from build123d import *

# Parameters (mm, degrees)
SKETCH_1_W          = 330
SKETCH_1_H          = 225
EXTRUDE_1_DEPTH     = 5
SKETCH_2_R          = 2
CUT_EXTRUDE_1_DEPTH = 395.101001153
SKETCH_3_R          = 2
CUT_EXTRUDE_2_DEPTH = 395.101001153
CUT_EXTRUDE_4_DEPTH = 395.101001153
SKETCH_6_R          = 2
CUT_EXTRUDE_5_DEPTH = 395.101001153


with BuildPart() as part:
    # 草图1 → 凸台-拉伸1 (new body)
    with BuildSketch(Plane(origin=(0, 0, 0), x_dir=(1, 0, 0), z_dir=(0, 1, 0))):
        with Locations((149.701456311, 124.678398058)):
            Rectangle(SKETCH_1_W, SKETCH_1_H)
    extrude(amount=EXTRUDE_1_DEPTH)

    # 草图2 → 切除-拉伸1 (cut, through all)
    with BuildSketch(Plane(origin=(0, 5, 0), x_dir=(1, 0, 0), z_dir=(0, 1, 0))):
        with Locations(Location((137.701456311, 230.178398058, 0), (0, 0, 270))):
            Circle(SKETCH_2_R)
        with Locations(Location((161.701456311, 230.178398058, 0), (0, 0, 90))):
            Circle(SKETCH_2_R)
        with Locations(Location((137.701456311, 212.178398058, 0), (0, 0, 270))):
            Circle(SKETCH_2_R)
        with Locations(Location((161.701456311, 212.178398058, 0), (0, 0, 90))):
            Circle(SKETCH_2_R)
        with BuildLine():
            Line((34.701456311, 225.715369926), (84.701456311, 225.715369926))
            ThreePointArc((84.701456311, 225.715369926), (89.238428179, 221.178398058), (84.701456311, 216.64142619))
            Line((84.701456311, 216.64142619), (34.701456311, 216.64142619))
            ThreePointArc((34.701456311, 216.64142619), (30.164484443, 221.178398058), (34.701456311, 225.715369926))
        make_face()
        with BuildLine():
            Line((264.701456311, 225.715369926), (214.701456311, 225.715369926))
            ThreePointArc((214.701456311, 225.715369926), (210.164484443, 221.178398058), (214.701456311, 216.64142619))
            Line((214.701456311, 216.64142619), (264.701456311, 216.64142619))
            ThreePointArc((264.701456311, 216.64142619), (269.238428179, 221.178398058), (264.701456311, 225.715369926))
        make_face()
    extrude(amount=-CUT_EXTRUDE_1_DEPTH, mode=Mode.SUBTRACT)

    # 草图3 → 切除-拉伸2 (cut, through all)
    with BuildSketch(Plane(origin=(0, 5, 0), x_dir=(1, 0, 0), z_dir=(0, 1, 0))):
        with Locations(Location((-0.298543689, 32.178398058, 0), (0, 0, 270))):
            Circle(SKETCH_3_R)
        with Locations(Location((-0.298543689, 72.178398058, 0), (0, 0, 90))):
            Circle(SKETCH_3_R)
        with Locations(Location((41.701456311, 32.178398058, 0), (0, 0, 270))):
            Circle(SKETCH_3_R)
        with Locations(Location((41.701456311, 72.178398058, 0), (0, 0, 90))):
            Circle(SKETCH_3_R)
        with Locations(Location((257.701456311, 72.178398058, 0), (0, 0, 270))):
            Circle(SKETCH_3_R)
        with Locations(Location((257.701456311, 32.178398058, 0), (0, 0, 90))):
            Circle(SKETCH_3_R)
        with Locations(Location((299.701456311, 72.178398058, 0), (0, 0, 270))):
            Circle(SKETCH_3_R)
        with Locations(Location((299.701456311, 32.178398058, 0), (0, 0, 90))):
            Circle(SKETCH_3_R)
    extrude(amount=-CUT_EXTRUDE_2_DEPTH, mode=Mode.SUBTRACT)

    # 草图5 → 切除-拉伸4 (cut, through all)
    with BuildSketch(Plane(origin=(0, 5, 0), x_dir=(1, 0, 0), z_dir=(0, 1, 0))):
        with BuildLine():
            Line((155.701456311, 161.411602286), (155.701456311, 61.411602286))
            ThreePointArc((155.701456311, 61.411602286), (149.701456311, 55.411602286), (143.701456311, 61.411602286))
            Line((143.701456311, 61.411602286), (143.701456311, 161.411602286))
            ThreePointArc((143.701456311, 161.411602286), (149.701456311, 167.411602286), (155.701456311, 161.411602286))
        make_face()
        with BuildLine():
            Line((239.701456311, 161.411602286), (239.701456311, 61.411602286))
            ThreePointArc((239.701456311, 61.411602286), (233.701456311, 55.411602286), (227.701456311, 61.411602286))
            Line((227.701456311, 61.411602286), (227.701456311, 161.411602286))
            ThreePointArc((227.701456311, 161.411602286), (233.701456311, 167.411602286), (239.701456311, 161.411602286))
        make_face()
        with BuildLine():
            Line((59.701456311, 161.411602286), (59.701456311, 61.411602286))
            ThreePointArc((59.701456311, 61.411602286), (65.701456311, 55.411602286), (71.701456311, 61.411602286))
            Line((71.701456311, 61.411602286), (71.701456311, 161.411602286))
            ThreePointArc((71.701456311, 161.411602286), (65.701456311, 167.411602286), (59.701456311, 161.411602286))
        make_face()
    extrude(amount=-CUT_EXTRUDE_4_DEPTH, mode=Mode.SUBTRACT)

    # 草图6 → 切除-拉伸5 (cut, through all)
    with BuildSketch(Plane(origin=(0, 5, 0), x_dir=(1, 0, 0), z_dir=(0, 1, 0))):
        with Locations(Location((1.226003167, 225.911661565, 0), (0, 0, 270))):
            Circle(SKETCH_6_R)
        with Locations(Location((298.176909455, 225.911661565, 0), (0, 0, 90))):
            Circle(SKETCH_6_R)
        with Locations(Location((69.701456311, 22.178398058, 0), (0, 0, 270))):
            Circle(SKETCH_6_R)
        with Locations(Location((229.701456311, 22.178398058, 0), (0, 0, 90))):
            Circle(SKETCH_6_R)
    extrude(amount=-CUT_EXTRUDE_5_DEPTH, mode=Mode.SUBTRACT)


solid = part.part
Verification items for the finished model (mm, model axes). A direction names the side the tool comes from. Coordinates: 2 decimals unless noted, no trailing zeros. Order: outer loops, then holes, each group sorted by start corner. A loop starts at its lowest first (then second) coordinate and runs counter-clockwise, first axis right, second up. Notation, with made-up numbers: M 61,38 L 76,38 A9 ccw 76,51 Z; hole C 0,7 d3. An arc over 180 degrees is marked long. Write each question's results on one line, items separated by ' | '.
1) Gauge pin test, flat end, axial feed: pin 1 Ø3 at (x, z) = (229.7, -22.18) entering from +Y. Record the tip position at first contact, or that the pin passes through.
Solved:
pin 1: passes through
2) Section check B-B on y = 1.3. Give the number of separate pieces and of enclosed holes in the cut face, plus the area to 3 significant figures.
Solved:
separate pieces: 1 | enclosed holes: 21 | area: 69,100 mm²
3) Access from +Z, -Z, +X, -X, +Y, -Y to the whole of each face (thin tool, end or side, straight path). Record for faces 1 (the face through (184, 0, -126)), 2 (the face through (65.83, 2.54, -167.41)).
Solved:
face 1: +Z, -Z, +X, -X, -Y | face 2: +Y, -Y
4) Scan lines: line 1 along X through (y, z) = (3.45, -117); line 2 along X through (y, z) = (0.65, -212.5); line 3 along Z through (x, y) = (237, 0.85). Record each from-to range of solid material in increasing order. Write a range as [from, to].
Solved:
line 1: x = [-15.3, 59.7], [71.7, 143.7], [155.7, 227.7], [239.7, 314.7] | line 2: x = [-15.3, 135.73], [139.68, 159.73], [163.68, 314.7] | line 3: z = [-237.18, -225.72], [-216.64, -166.42], [-56.4, -12.18]
5) Section check A-A on z = -81. Record the cut outline in (x, y), plus the area to 3 significant figures.
Solved:
outline: M -15.3,0 L 59.7,0 L 59.7,5 L -15.3,5 Z; M 71.7,0 L 143.7,0 L 143.7,5 L 71.7,5 Z; M 155.7,0 L 227.7,0 L 227.7,5 L 155.7,5 Z; M 239.7,0 L 314.7,0 L 314.7,5 L 239.7,5 Z | area: 1,470 mm²
6) Release check for a two-part mould opening along Z. For faces 3 (the face through (233.833, 2.535, -55.413)), 4 (the face through (184, 5, -126)), 5 (the face through (233.57, 2.54, -167.41)) record: pulls with the +Z half, pulls with the -Z half, needs draft (parallel to the pull), parting line crosses it, or undercut.
Solved:
face 3: undercut | face 4: needs draft | face 5: undercut
